from build123d import *

# Parameters (mm, degrees)
SKETCH1_W           = 15
SKETCH1_H           = 12.5
BOSS_EXTRUDE1_DEPTH = 6.5
SKETCH2_R           = 1.5
CUT_EXTRUDE1_DEPTH  = 12.728704106
CHAMFER1_SIZE       = 3.4
CHAMFER1_SIZE2      = 8.009898044
SKETCH2_3_R         = 2.5
SKETCH2_3_R_2       = 1.5
CUT_EXTRUDE5_DEPTH  = 1.2
CUT_EXTRUDE4_DEPTH  = 5.25
SKETCH3_W           = 5.5
SKETCH3_H           = 2
CUT_EXTRUDE3_DEPTH  = 3.25
CHAMFER2_SIZE       = 1.5


with BuildPart() as part:
    # Sketch1 → Boss-Extrude1 (new body)
    with BuildSketch(Plane(origin=(0, 0, 0), x_dir=(1, 0, 0), z_dir=(0, 1, 0))):
        Rectangle(SKETCH1_W, SKETCH1_H)
    extrude(amount=BOSS_EXTRUDE1_DEPTH)

    # Sketch2 → Cut-Extrude1 (cut, through all)
    with BuildSketch(Plane(origin=(0, 0, 0), x_dir=(1, 0, 0), z_dir=(0, 1, 0))):
        with Locations(Location((4.75, 1, 0), (0, 0, 90))):
            Circle(SKETCH2_R)
        with Locations(Location((-4.75, 1, 0), (0, 0, 90))):
            Circle(SKETCH2_R)
    extrude(amount=CUT_EXTRUDE1_DEPTH, mode=Mode.SUBTRACT)

    # Chamfer1
    chamfer1_edges = [part.edges().sort_by_distance(p)[0] for p in [
        (7.5, 3.25, 6.25),
        (-7.5, 3.25, 6.25),
    ]]
    chamfer1_side = [part.faces().sort_by_distance(p)[0] for p in [
        (0, 3.25, 6.25),
    ]]
    chamfer(chamfer1_edges, length=CHAMFER1_SIZE, length2=CHAMFER1_SIZE2, reference=chamfer1_side[0])

    # Sketch2<3> → Cut-Extrude5 (cut)
    # profile 1 of 2: a face of its own
    with BuildSketch(Plane(origin=(0, 0, 0), x_dir=(1, 0, 0), z_dir=(0, 1, 0))):
        with Locations((4.75, 1)):
            Circle(SKETCH2_3_R)
        with Locations(Location((4.75, 1, 0), (0, 0, 90))):
            Circle(SKETCH2_3_R_2, mode=Mode.SUBTRACT)
    # profile 2 of 2: a face of its own
    with BuildSketch(Plane(origin=(0, 0, 0), x_dir=(1, 0, 0), z_dir=(0, 1, 0))):
        with Locations((-4.75, 1)):
            Circle(SKETCH2_3_R)
        with Locations(Location((-4.75, 1, 0), (0, 0, 90))):
            Circle(SKETCH2_3_R_2, mode=Mode.SUBTRACT)
    extrude(amount=CUT_EXTRUDE5_DEPTH, mode=Mode.SUBTRACT)

    # Sketch3<3> → Cut-Extrude4 (cut)
    with BuildSketch(Plane(origin=(0, 6.5, 0), x_dir=(1, 0, 0), z_dir=(0, 1, 0))):
        Polygon((7.5, 4.75), (-7.5, 4.75), (-7.5, 3.25), (-2.75, 3.25), (2.75, 3.25), (7.5, 3.25), align=None)
    extrude(amount=-CUT_EXTRUDE4_DEPTH, mode=Mode.SUBTRACT)

    # Sketch4 → Cut-Revolve1 (revolve, cut)
    with BuildSketch(Plane(origin=(0, 6.5, 0), x_dir=(1, 0, 0), z_dir=(0, 1, 0))):
        Polygon((2.75, 1.25), (2.75, -0.5), (1.75, -0.5), (2.75, -2), (2.75, -4.75), (1.75, -4.75), (2.75, -6.25), (0, -6.25), (0, 1.25), align=None)
    revolve(axis=Axis((0, 6.5, 6.25), (0, 0, -1)), mode=Mode.SUBTRACT)

    # Sketch3 → Cut-Extrude3 (cut)
    with BuildSketch(Plane(origin=(0, 6.5, 0), x_dir=(1, 0, 0), z_dir=(0, 1, 0))):
        with Locations((0, 2.25)):
            Rectangle(SKETCH3_W, SKETCH3_H)
    extrude(amount=-CUT_EXTRUDE3_DEPTH, mode=Mode.SUBTRACT)

    # Chamfer2
    chamfer2_edges = [part.edges().sort_by_distance(p)[0] for p in [
        (-7.5, 3.25, -6.25),
        (7.5, 3.25, -6.25),
    ]]
    chamfer(chamfer2_edges, length=CHAMFER2_SIZE - 0.0001)  # a hair under: the kernel refuses the full size


solid = part.part
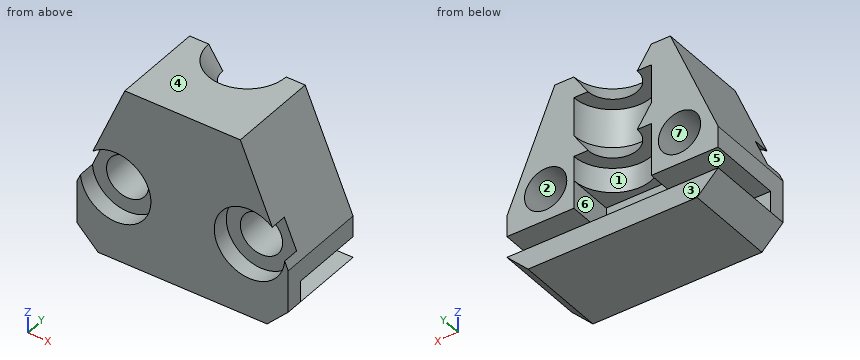
Design review of the part built by this model. Coordinates are the model's own, in mm. Face numbers are marked on the shaded views. A direction names the side the tool comes from. Give positions to 0.01 mm unless a question says otherwise; leave off trailing zeros. Loops run counter-clockwise (first coordinate to the right, second up) from the corner with the lowest first, then second, coordinate; pieces in that order, holes last. Notation, with made-up numbers: (-34, 14.25) -> (-30, 14.25) arc R21 cw to (-30, 51.25) -> close; hole circle Ø7 at (71, 54.5). An arc over 180 degrees is marked (long way). One line per question, with ' | ' between items. Start each with the question number.
(1) Insertion check: P1, Ø1.5, axis at x = -5, z = -0.5, coming from the -Y side (3 decimals); P2, Ø1.6, axis at x = -1, z = -2.5, coming from the +Y side. Each pin has a flat end and moves straight along its axis. Give the tip position at first contact, or say it passes through.
(2) Draft analysis for pull direction Z (two halves, no side actions). For the marked faces 1, 2, 3 and 4, state which applies: +Z half, -Z half, draft (parallel to the pull), parting line (faces both ways), or undercut.
(3) For the marked faces 5, 6 and 7, list the 3-axis set-ups (+Z, -Z, +X, -X, +Y, -Y) from which the entire face can be reached by the end or side of a thin tool; tool diameter is ignored.
(4) We need section B-B (x = -4.5). State the section outline as (y, z) points.
(5) We need section C-C (z = 0.25). State the section outline as (x, y) points.
(6) For line 1 (Z direction, x = 4.75, y = 5.45); line 2 (X direction, y = 3, z = -1.75); line 3 (Z direction, x = -5, y = 2.75), list the stretches that pass through material, from the lowest coordinate up.
(7) We need section A-A (y = 2). State how many separate pieces and enclosed holes the cut face has, and give its area (3 significant figures).
(8) We need section D-D (x = 0). State the section outline as (y, z) points, and give its area (4 significant figures).
The answers:
1) P1: passes through | P2: stops at y = 3.25
2) face 1: undercut | face 2: undercut | face 3: draft | face 4: +Z half
3) face 5: +X, -X, +Y | face 6: +Y | face 7: +Y, -Y
4) outline: (0, -6.25) -> (6.5, -6.25) -> (6.5, -4.75) -> (1.25, -4.75) -> (1.25, -3.25) -> (6.5, -3.25) -> (6.5, -2.48) -> (1.2, -2.48) -> (1.2, -3.49) -> (0, -3.49) -> close; (0, 1.49) -> (1.2, 1.49) -> (1.2, 0.48) -> (6.5, 0.48) -> (6.5, 5.31) -> (0, 5.31) -> close
5) outline: (-6.65, 1.2) -> (-5.58, 1.2) -> (-5.58, 6.5) -> (-6.65, 6.5) -> close; (-3.92, 1.2) -> (-2.58, 1.2) -> (-2.58, 0) -> (2.58, 0) -> (2.58, 1.2) -> (3.92, 1.2) -> (3.92, 6.5) -> (2.75, 6.5) arc R2.75 cw to (-2.75, 6.5) -> (-3.92, 6.5) -> close; (5.58, 1.2) -> (6.65, 1.2) -> (6.65, 6.5) -> (5.58, 6.5) -> close
6) line 1: z = -6.25 to -4.75, -3.25 to -2.5, 0.5 to 4.72 | line 2: x = -7.5 to -6.05, -3.45 to 3.45, 6.05 to 7.5 | line 3: z = -6.25 to -4.75, -3.25 to -2.48, 0.48 to 4.13
7) separate pieces: 2 | enclosed holes: 2 | area: 121 mm^2
8) outline: (0, -6.25) -> (6.5, -6.25) -> (6.5, -4.75) -> (1.25, -4.75) -> (1.25, -3.25) -> (3.25, -3.25) -> (3.25, -1.25) -> (3.75, -1.25) -> (3.75, 0.5) -> (4.75, 0.5) -> (3.75, 2) -> (3.75, 4.75) -> (4.75, 4.75) -> (3.75, 6.25) -> (0, 6.25) -> close | area: 47.75 mm^2
